Check sheet for the drawn part. Datum: minimum x, y, z corner. Units: mm. A direction names the side the tool comes from. Give positions to 0.01 mm unless a question says otherwise; leave off trailing zeros. Loops run counter-clockwise (first coordinate to the right, second up) from the corner with the lowest first, then second, coordinate; pieces in that order, holes last.
1. Material ranges on L1, parallel to Z at x = 7.5, y = 1.75; L2, parallel to Y at x = 2.25, z = 6.75; L3, parallel to Y at x = 6.25, z = 5.5, recorded low to high.
2. Cross-section at D-D, the plane z = 5.25. Record the cut outline in (x, y), plus the area to 3 significant figures.
3. Go/stop test with flat-tipped pins: pin 1 Ø0.9 at (x, z) = (3, 7) entering from +Y; pin 2 Ø0.6 at (y, z) = (2.5, 7) entering from +X; pin 3 Ø2 at (y, z) = (3.5, 3) entering from -X. Record where each tip stops, or that it passes through.
4. Cross-section at C-C, the plane z = 0.5. Record the cut outline in (x, y).
5. Tool access check on the marked faces 1 and 2. Record the directions out of +Z, -Z, +X, -X, +Y, -Y that give a thin tool (end or side, any length) a straight path to the whole face; none if there is none.
6. Cross-section at A-A, the plane y = 5. Record the cut outline in (x, z), plus the area to 3 significant figures.
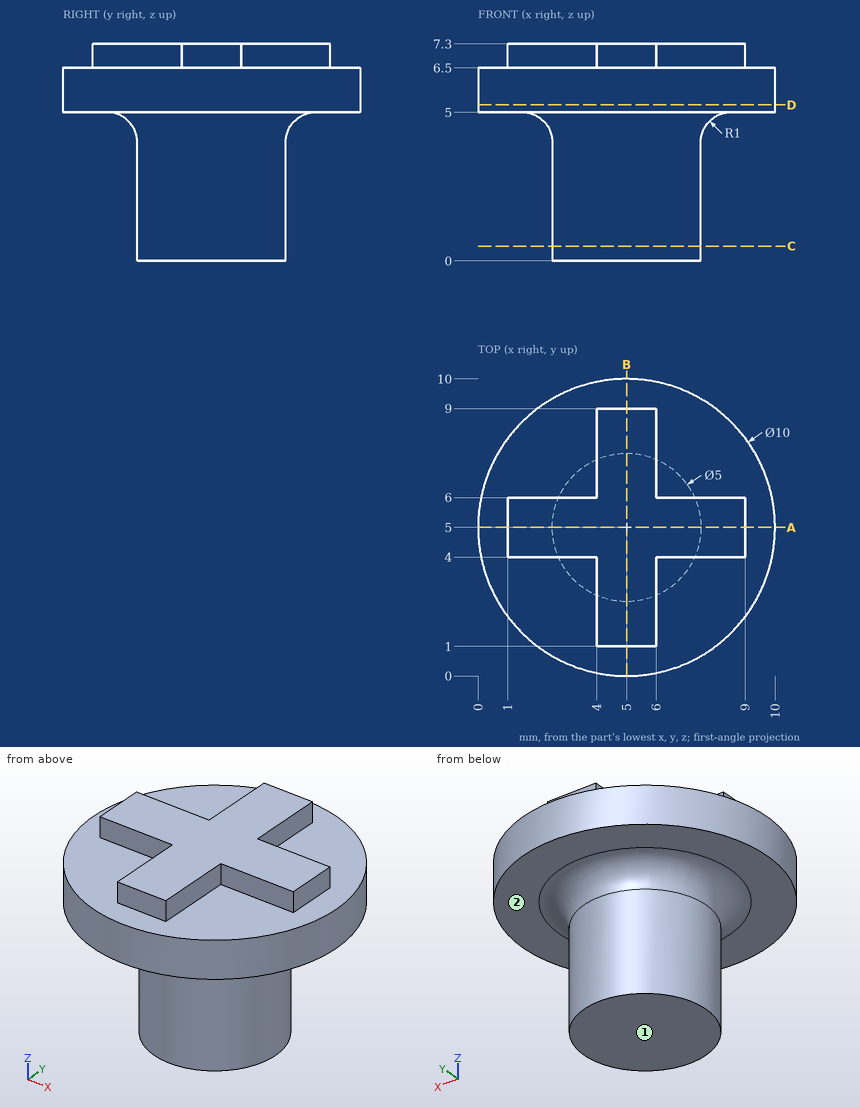
Result:
1. L1: z = 5 to 6.5
1. L2: y = 4 to 6
1. L3: y = 0.16 to 9.84
2. outline: circle Ø10 at (5, 5)
2. area: 78.5 mm2
3. pin 1: stops at y = 6
3. pin 2: stops at x = 6
3. pin 3: stops at x = 2.55
4. outline: circle Ø5 at (5, 5)
5. face 1: -Z, +X, -X, +Y, -Y
5. face 2: -Z
6. outline: (0, 5) - (1.5, 5) arc R1 cw to (2.5, 4) - (2.5, 0) - (7.5, 0) - (7.5, 4) arc R1 cw to (8.5, 5) - (10, 5) - (10, 6.5) - (9, 6.5) - (9, 7.3) - (1, 7.3) - (1, 6.5) - (0, 6.5) - close
6. area: 46.8 mm2
